For this review, take the finished solid that the model builds, in its own axes (mm). Give positions to 0.01 mm unless a question says otherwise; leave off trailing zeros. Order: outer loops, then holes, each group sorted by start corner. A loop starts at its lowest first (then second) coordinate and runs counter-clockwise, first axis right, second up.
from build123d import *


with BuildPart() as part:
    # Sketch1 → Revolve1 (revolve)
    with BuildSketch(Plane.XZ):
        with BuildLine():
            Line((10, 223), (0, 223))
            Line((0, 223), (0, 63))
            Line((0, 63), (10, 63))
            ThreePointArc((10, 63), (10.878679656, 60.878679656), (13, 60))
            Line((13, 60), (13.5, 60))
            ThreePointArc((13.5, 60), (15.621320344, 60.878679656), (16.5, 63))
            Line((16.5, 63), (16.5, 67))
            ThreePointArc((16.5, 67), (15.621320344, 69.121320344), (13.5, 70))
            Line((13.5, 70), (10, 70))
            Line((10, 70), (10, 223))
        make_face()
    revolve(axis=Axis((0, 0, 223), (0, 0, -1)))


solid = part.part
1) We need section C-C on z = 175. Give the boundary of the cut face in (x, y), then the cut area to 3 significant figures.
Answer sheet:
outline: circle Ø20 at (0, 0)
area: 314 mm2
2) We need section A-A on x = 0. Give the boundary of the cut face in (y, z).
Answer sheet:
outline: (-16.5, 63) arc R3 ccw to (-13.5, 60) - (-13, 60) arc R3 ccw to (-10, 63) - (10, 63) arc R3 ccw to (13, 60) - (13.5, 60) arc R3 ccw to (16.5, 63) - (16.5, 67) arc R3 ccw to (13.5, 70) - (10, 70) - (10, 223) - (-10, 223) - (-10, 70) - (-13.5, 70) arc R3 ccw to (-16.5, 67) - close
3) Draft analysis for pull direction Y (two halves, no side actions). For faces 1 (the face through (-2.17, 9.76, 147.57)), 2 (the face through (-9, 5, 70)), 3 (the face through (0, 0, 63)), state which applies: +Y half, -Y half, draft (parallel to the pull), parting line (faces both ways), or undercut.
Answer sheet:
face 1: parting line
face 2: draft
face 3: undercut
4) Clearance check with flat-ended pins moving along their axes: pin 1 (3 mm diameter, centred on y = 0, z = 143, fed in from +X); pin 2 (8 mm diameter, centred on x = -6, z = 170.5, fed in from +Y); pin 3 (6 mm diameter, centred on y = 8.5, z = 118.5, fed in from -X). State where each tip first meets the part, or that it passes through.
Answer sheet:
pin 1: stops at x = 10
pin 2: stops at y = 9.8
pin 3: stops at x = -8.35
5) To check wall thickness, follow line 1 (Y direction, x = 0, z = 123); line 2 (Z direction, x = -2, y = 13). State the ranges of each line that lie inside material, in increasing order.
Answer sheet:
line 1: y = -10 to 10
line 2: z = 60 to 70
